```python
from build123d import *

# Parameters (mm, degrees)
BOSS_EXTRUDE1_DEPTH = 381
SKETCH2_R           = 31.75
SKETCH2_W           = 27.94
SKETCH2_H           = 27.94
CUT_EXTRUDE2_DEPTH  = 15.24
SKETCH2_3_W         = 27.94
SKETCH2_3_H         = 27.94
CUT_EXTRUDE3_DEPTH  = 43.18
SHELL1_T            = -3.81


with BuildPart() as part:
    # Sketch1 → Boss-Extrude1 (new body)
    with BuildSketch(Plane(origin=(0, 0, 0), x_dir=(0, 0, -1), z_dir=(1, 0, 0))):
        Polygon((0, 0), (0, 38.1), (302.409374855, 76.2), (302.409374855, 0), align=None)
    extrude(amount=BOSS_EXTRUDE1_DEPTH)

    # Sketch2 → Cut-Extrude2 (cut)
    # profile 1 of 9: a face of its own
    with BuildSketch(Plane(origin=(0, 40.024765624, 5.042646482), x_dir=(1, 0, 0), z_dir=(0, 0.9921567416492215, 0.12500000000000003))):
        with Locations(Location((63.5, 246.0625, 0), (0, 0, 270))):
            Circle(SKETCH2_R)
        with Locations((63.5, 246.0625)):
            Rectangle(SKETCH2_W, SKETCH2_H, mode=Mode.SUBTRACT)
    # profile 2 of 9: a face of its own
    with BuildSketch(Plane(origin=(0, 40.024765624, 5.042646482), x_dir=(1, 0, 0), z_dir=(0, 0.9921567416492215, 0.12500000000000003))):
        with Locations(Location((190.5, 246.0625, 0), (0, 0, 270))):
            Circle(SKETCH2_R)
        with Locations((190.5, 246.0625)):
            Rectangle(SKETCH2_W, SKETCH2_H, mode=Mode.SUBTRACT)
    # profile 3 of 9: a face of its own
    with BuildSketch(Plane(origin=(0, 40.024765624, 5.042646482), x_dir=(1, 0, 0), z_dir=(0, 0.9921567416492215, 0.12500000000000003))):
        with Locations(Location((317.5, 246.0625, 0), (0, 0, 270))):
            Circle(SKETCH2_R)
        with Locations((317.5, 246.0625)):
            Rectangle(SKETCH2_W, SKETCH2_H, mode=Mode.SUBTRACT)
    # profile 4 of 9: a face of its own
    with BuildSketch(Plane(origin=(0, 40.024765624, 5.042646482), x_dir=(1, 0, 0), z_dir=(0, 0.9921567416492215, 0.12500000000000003))):
        with Locations(Location((63.5, 157.1625, 0), (0, 0, 270))):
            Circle(SKETCH2_R)
        with Locations((63.5, 157.1625)):
            Rectangle(SKETCH2_W, SKETCH2_H, mode=Mode.SUBTRACT)
    # profile 5 of 9: a face of its own
    with BuildSketch(Plane(origin=(0, 40.024765624, 5.042646482), x_dir=(1, 0, 0), z_dir=(0, 0.9921567416492215, 0.12500000000000003))):
        with Locations(Location((63.5, 68.2625, 0), (0, 0, 270))):
            Circle(SKETCH2_R)
        with Locations((63.5, 68.2625)):
            Rectangle(SKETCH2_W, SKETCH2_H, mode=Mode.SUBTRACT)
    # profile 6 of 9: a face of its own
    with BuildSketch(Plane(origin=(0, 40.024765624, 5.042646482), x_dir=(1, 0, 0), z_dir=(0, 0.9921567416492215, 0.12500000000000003))):
        with Locations(Location((190.5, 157.1625, 0), (0, 0, 270))):
            Circle(SKETCH2_R)
        with Locations((190.5, 157.1625)):
            Rectangle(SKETCH2_W, SKETCH2_H, mode=Mode.SUBTRACT)
    # profile 7 of 9: a face of its own
    with BuildSketch(Plane(origin=(0, 40.024765624, 5.042646482), x_dir=(1, 0, 0), z_dir=(0, 0.9921567416492215, 0.12500000000000003))):
        with Locations(Location((190.5, 68.2625, 0), (0, 0, 270))):
            Circle(SKETCH2_R)
        with Locations((190.5, 68.2625)):
            Rectangle(SKETCH2_W, SKETCH2_H, mode=Mode.SUBTRACT)
    # profile 8 of 9: a face of its own
    with BuildSketch(Plane(origin=(0, 40.024765624, 5.042646482), x_dir=(1, 0, 0), z_dir=(0, 0.9921567416492215, 0.12500000000000003))):
        with Locations(Location((317.5, 68.2625, 0), (0, 0, 270))):
            Circle(SKETCH2_R)
        with Locations((317.5, 68.2625)):
            Rectangle(SKETCH2_W, SKETCH2_H, mode=Mode.SUBTRACT)
    # profile 9 of 9: a face of its own
    with BuildSketch(Plane(origin=(0, 40.024765624, 5.042646482), x_dir=(1, 0, 0), z_dir=(0, 0.9921567416492215, 0.12500000000000003))):
        with Locations(Location((317.5, 157.1625, 0), (0, 0, 270))):
            Circle(SKETCH2_R)
        with Locations((317.5, 157.1625)):
            Rectangle(SKETCH2_W, SKETCH2_H, mode=Mode.SUBTRACT)
    extrude(amount=-CUT_EXTRUDE2_DEPTH, mode=Mode.SUBTRACT)

    # Sketch2_3 → Cut-Extrude3 (cut)
    with BuildSketch(Plane(origin=(0, 40.024765624, 5.042646482), x_dir=(1, 0, 0), z_dir=(0, 0.9921567416492215, 0.12500000000000003))):
        with Locations((63.5, 68.2625)):
            Rectangle(SKETCH2_3_W, SKETCH2_3_H)
        with Locations((63.5, 157.1625)):
            Rectangle(SKETCH2_3_W, SKETCH2_3_H)
        with Locations((63.5, 246.0625)):
            Rectangle(SKETCH2_3_W, SKETCH2_3_H)
        with Locations((190.5, 246.0625)):
            Rectangle(SKETCH2_3_W, SKETCH2_3_H)
        with Locations((190.5, 157.1625)):
            Rectangle(SKETCH2_3_W, SKETCH2_3_H)
        with Locations((190.5, 68.2625)):
            Rectangle(SKETCH2_3_W, SKETCH2_3_H)
        with Locations((317.5, 157.1625)):
            Rectangle(SKETCH2_3_W, SKETCH2_3_H)
        with Locations((317.5, 68.2625)):
            Rectangle(SKETCH2_3_W, SKETCH2_3_H)
        with Locations((317.5, 246.0625)):
            Rectangle(SKETCH2_3_W, SKETCH2_3_H)
    extrude(amount=-CUT_EXTRUDE3_DEPTH, mode=Mode.SUBTRACT)

    # Shell1
    shell1_openings = [part.faces().sort_by_distance(p)[0] for p in [
        (190.5, 0, -151.204687427),
    ]]
    offset(amount=SHELL1_T, openings=shell1_openings, kind=Kind.INTERSECTION)


solid = part.part
```
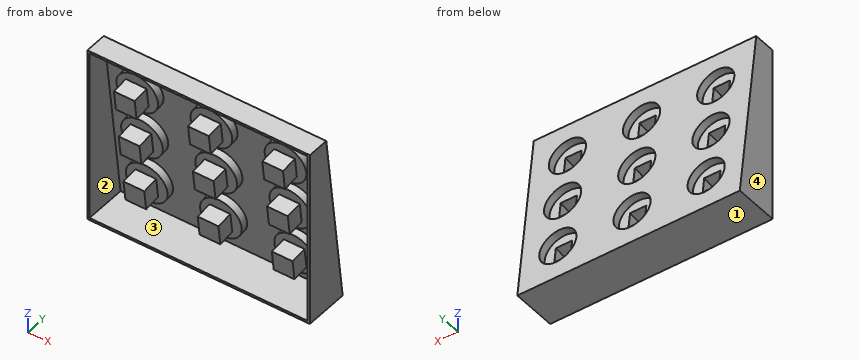
Check sheet for the modelled part. Datum: model origin and axes. Units: mm. Face numbers are marked on the shaded views. Round coordinates to 2 decimals unless told otherwise and drop trailing zeros. Order: outer loops, then holes, each group sorted by start corner. A loop starts at its lowest first (then second) coordinate and runs counter-clockwise, first axis right, second up. Notation, with made-up numbers: (9.5, 73.5) - (60.5, 73.5) arc R16 cw to (60.5, 84.5) - close; hole circle Ø11 at (-5, 2.25). An arc over 180 degrees is marked (long way). Answer as CSV lines item,"result". Start each with the question number.
1) Section check B-B (x = 103). Record the cut outline in (y, z), then the cut area to 3 significant figures.
2) Draft check along Z on the marked faces 1, 2, 3 and 4. Enter one of: +Z half, -Z half, draft (parallel to the pull), parting line (faces both ways), or undercut.
3) Depth check by flat-ended pin: pin 1 (12 mm diameter, centred on x = 286, z = -194, fed in from -Y); pin 2 (10 mm diameter, centred on x = 65, z = -239, fed in from -Y); pin 3 (2 mm diameter, centred on x = 262, z = -75, fed in from -Y). Enter the tip coordinate at first touch or a pass-through.
4) Scan lines: probe 1 along X at (y, z) = (10.5, -215); probe 2 along Z at (x, y) = (294, 6.5); probe 3 along Z at (x, y) = (204.5, 7). Record each from-to range of solid material in increasing order.
Determined:
1,outline,"(0, -302.41) - (76.2, -302.41) - (38.1, 0) - (0, 0) - (0, -3.81) - (34.74, -3.81) - (71.88, -298.6) - (0, -298.6) - close"
1,area,"1,570 mm^2"
2,face 1,"-Z half"
2,face 2,"undercut"
2,face 3,"undercut"
2,face 4,"draft"
3,pin 1,"y = 57.95"
3,pin 2,"y = 22.78"
3,pin 3,"y = 43.58"
4,probe 1,"0 to 3.81, 377.19 to 381"
4,probe 2,"-302.41 to -298.6, -3.81 to 0"
4,probe 3,"-302.41 to -298.6, -85.84 to -50, -3.81 to 0"
